Here's how the part is built. I have some questions about the finished solid (model axes, mm). A direction names the side the tool comes from. Give positions to 0.01 mm unless a question says otherwise; leave off trailing zeros. Write each loop counter-clockwise with the first axis right and the second up, starting at its lowest first coordinate (ties: lowest second). Pieces come first, ordered by that corner, then holes. Notation, with made-up numbers: (-25, 27) -> (31, 27) arc R24 ccw to (31, 51) -> close; hole circle Ø6 at (25.25, 41.25). An arc over 180 degrees is marked (long way). Use one line per item in the form item = value.
```python
from build123d import *

# Parameters (mm, degrees)
BASE_FLANGE1_DEPTH = 5
SKETCH17_R         = 5
CUT_EXTRUDE1_DEPTH = 2.5
SKETCH39_R         = 2.5
CUT_EXTRUDE2_DEPTH = 10
CUT_EXTRUDE4_DEPTH = 59.202233634
SKETCH40_R         = 5
SKETCH40_R_2       = 2.5
CUT_EXTRUDE6_DEPTH = 2.5


# Sheet-metal steps are written as plain solids
with BuildPart() as part:
    # Sketch1 → Base-Flange1 (new body)
    with BuildSketch(Plane.XY):
        with BuildLine():
            Line((0, 7.5), (50, 7.5))
            ThreePointArc((50, 7.5), (57.5, 0), (50, -7.5))
            Line((50, -7.5), (0, -7.5))
            ThreePointArc((0, -7.5), (-7.5, 0), (0, 7.5))
        make_face()
    extrude(amount=-BASE_FLANGE1_DEPTH)

    # Sketch17 → Cut-Extrude1 (cut)
    with BuildSketch(Plane(origin=(0, 0, -5), x_dir=(-1, 0, 0), z_dir=(0, 0, -1))):
        Circle(SKETCH17_R)
    extrude(amount=-CUT_EXTRUDE1_DEPTH, mode=Mode.SUBTRACT)

    # Sketch39 → Cut-Extrude2 (cut)
    with BuildSketch(Plane.XY):
        Circle(SKETCH39_R)
        with Locations((50, 0)):
            Circle(SKETCH39_R)
    extrude(amount=-CUT_EXTRUDE2_DEPTH, mode=Mode.SUBTRACT)

    # Sketch41 → Cut-Extrude4 (cut, through all)
    with BuildSketch(Plane.XY):
        with BuildLine():
            Line((25, 2.5), (50, 2.5))
            ThreePointArc((50, 2.5), (52.5, 0), (50, -2.5))
            Line((50, -2.5), (25, -2.5))
            ThreePointArc((25, -2.5), (22.5, 0), (25, 2.5))
        make_face()
    extrude(amount=-CUT_EXTRUDE4_DEPTH, mode=Mode.SUBTRACT)

    # Sketch40 → Cut-Extrude6 (cut)
    # profile 1 of 2: a face of its own
    with BuildSketch(Plane.XY):
        with Locations((50, 0)):
            Circle(SKETCH40_R)
        with Locations((50, 0)):
            Circle(SKETCH40_R_2, mode=Mode.SUBTRACT)
    # profile 2 of 2: a face of its own
    with BuildSketch(Plane.XY):
        with BuildLine():
            Line((25, -5), (50, -5))
            ThreePointArc((50, -5), (45, 0), (50, 5))
            Line((50, 5), (25, 5))
            ThreePointArc((25, 5), (20, 0), (25, -5))
        make_face()
    extrude(amount=-CUT_EXTRUDE6_DEPTH, mode=Mode.SUBTRACT)


solid = part.part
```
Q1. If we mould it in two halves opening along X, with no side actions, what happens to faces 1 (the face through (-7.5, -0.16, -2.46)), 2 (the face through (37, -5, -1)), 3 (the face through (18, 0, 0)), 4 (the face through (57.5, 0.16, -2.46))? For each: +X half, -X half, draft (parallel to the pull), parting line (faces both ways), or undercut.
Result set:
face_1 = -X half
face_2 = undercut
face_3 = draft
face_4 = +X half
Q2. I want a section at B-B, the plane x = 35. Write out the boundary of the cut face in (y, z), and give its area (3 significant figures).
Result set:
outline = (-7.5, -5) -> (-2.5, -5) -> (-2.5, -2.5) -> (-5, -2.5) -> (-5, 0) -> (-7.5, 0) -> close; (2.5, -5) -> (7.5, -5) -> (7.5, 0) -> (5, 0) -> (5, -2.5) -> (2.5, -2.5) -> close
area = 37.5 mm2
Q3. I want a section at C-C, the plane y = 0. Write out the boundary of the cut face in (x, z).
Result set:
outline = (-7.5, -5) -> (-5, -5) -> (-5, -2.5) -> (-2.5, -2.5) -> (-2.5, 0) -> (-7.5, 0) -> close; (2.5, -2.5) -> (5, -2.5) -> (5, -5) -> (22.5, -5) -> (22.5, -2.5) -> (20, -2.5) -> (20, 0) -> (2.5, 0) -> close; (52.5, -5) -> (57.5, -5) -> (57.5, 0) -> (55, 0) -> (55, -2.5) -> (52.5, -2.5) -> close
Q4. I want a section at A-A, the plane z = -0.55. Write out the boundary of the cut face in (x, y), and give its area (3 significant figures).
Result set:
outline = (0, -7.5) -> (50, -7.5) arc R7.5 ccw to (50, 7.5) -> (0, 7.5) arc R7.5 ccw to start; hole circle Ø5 at (0, 0); hole (25, -5) -> (50, -5) arc R5 ccw to (50, 5) -> (25, 5) arc R5 ccw to start
area = 579 mm2
Q5. Which directions (+Z, -Z, +X, -X, +Y, -Y) give clear straight access to the entire face, cutting with the end or side of a thin tool? Please do faces 5 (the face through (22.5, -0.1, -3.7)), 6 (the face through (1.08, -4.88, -3.77)), 7 (the face through (25, -7.5, -2)), 8 (the face through (38, 5, -1)), 9 (the face through (25, 7.5, -2)).
Result set:
face_5 = +Z, -Z
face_6 = -Z
face_7 = +Z, -Z, +X, -X, -Y
face_8 = +Z
face_9 = +Z, -Z, +X, -X, +Y
Q6. I want a section at D-D, the plane z = -4.35. Write out the boundary of the cut face in (x, y), and give its area (3 significant figures).
Result set:
outline = (0, -7.5) -> (50, -7.5) arc R7.5 ccw to (50, 7.5) -> (0, 7.5) arc R7.5 ccw to start; hole circle Ø10 at (0, 0); hole (25, -2.5) -> (50, -2.5) arc R2.5 ccw to (50, 2.5) -> (25, 2.5) arc R2.5 ccw to start
area = 704 mm2
Q7. If I drill on line 1 along X through (y, z) = (1.5, -3.7); line 2 along Y through (x, z) = (0, -0.9); line 3 along Y through (x, z) = (0, -4.25), over which ranges is the centre line in solid material (lowest first)? Write a range as from..to.
Result set:
line_1 = -7.35..-4.77, 4.77..23, 52..57.35
line_2 = -7.5..-2.5, 2.5..7.5
line_3 = -7.5..-5, 5..7.5
